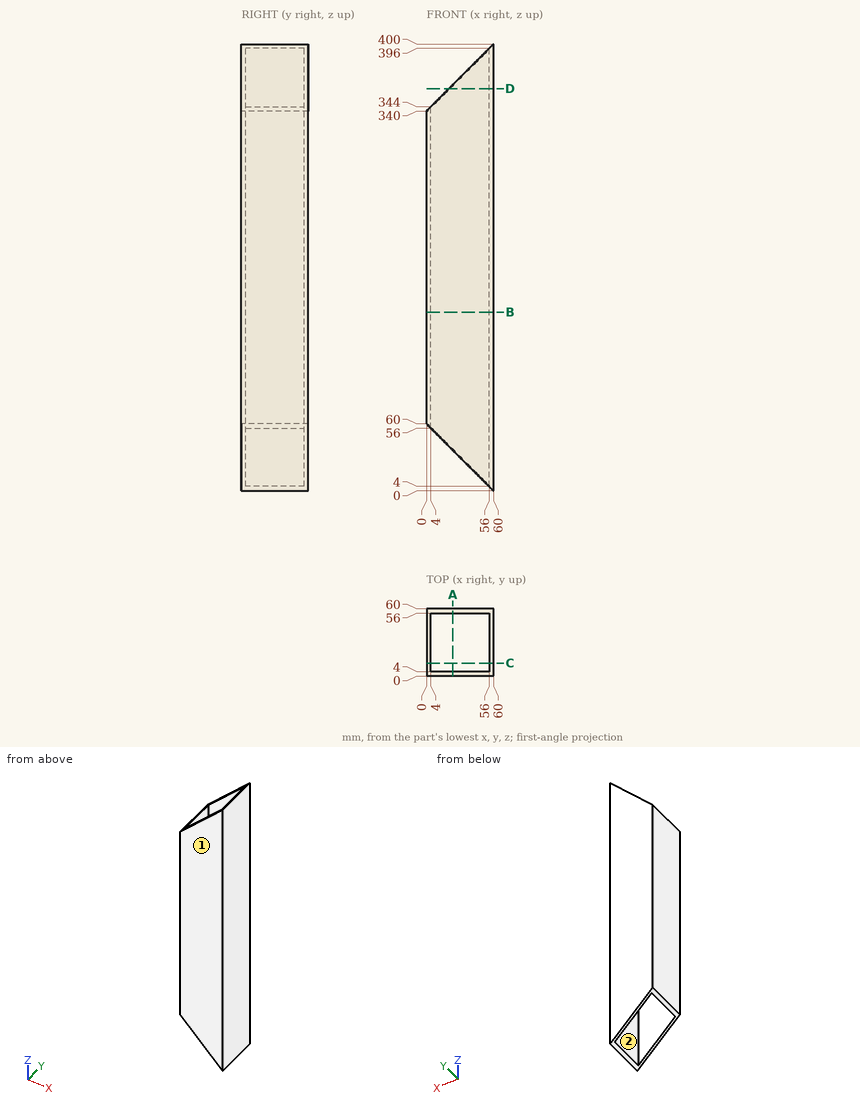
Job drawing, mm, ordinate dimensions from the low corner. One solid piece. A direction names the side the tool comes from. Give positions to 0.01 mm unless a question says otherwise; leave off trailing zeros. Loops run counter-clockwise (first coordinate to the right, second up) from the corner with the lowest first, then second, coordinate; pieces in that order, holes last. Notation, with made-up numbers: M -1,52 L 37,52 A26 ccw 37,71 Z; hole C 3.5,8.5 d9. An arc over 180 degrees is marked long. Return JSON: item names as keys, results as strings.
1) Saw through at C-C, the plane y = 11.5. List the corners of the cut face in (x, z).
Calculated:
{"outline": "M 0,60 L 4,56 L 4,344 L 0,340 Z; M 56,4 L 60,0 L 60,400 L 56,396 Z"}
2) Saw through at D-D, the plane z = 360. List the corners of the cut face in (x, y), then the cut area to 3 significant figures.
Calculated:
{"outline": "M 20,0 L 60,0 L 60,60 L 20,60 L 20,56 L 56,56 L 56,4 L 20,4 Z", "area": "528 mm2"}
3) Saw through at A-A, the plane x = 23.5. List the corners of the cut face in (y, z).
Calculated:
{"outline": "M 0,36.5 L 4,36.5 L 4,363.5 L 0,363.5 Z; M 56,36.5 L 60,36.5 L 60,363.5 L 56,363.5 Z"}
4) 3-axis set-ups, long thin cutter, end or side, ignore diameter. For the marked faces 1 and 2: which of +Z, -Z, +X, -X, +Y, -Y reach the whole face in a straight line?
Calculated:
{"face 1": "+Z, -Z, +X, -X, -Y", "face 2": "+Z, -Z"}
5) Saw through at B-B, the plane z = 160. List the corners of the cut face in (x, y), then the cut area to 3 significant figures.
Calculated:
{"outline": "M 0,0 L 60,0 L 60,60 L 0,60 Z; hole M 4,4 L 56,4 L 56,56 L 4,56 Z", "area": "896 mm2"}
6) Drill centre lines: line 1 (Y direction, x = 22.5, z = 270); line 2 (X direction, y = 16, z = 346). Where is each one in solid material? Low to high.
Calculated:
{"line 1": "y = 0 to 4, 56 to 60", "line 2": "x = 56 to 60"}
7) Flat gauge pin, fed straight in: pin 1 Ø8 at (x, y) = (9, 50) entering from -Z. Where does the tip first touch, or does it go through?
Calculated:
{"pin 1": "passes through"}
